Here's how the part is built. I have some questions about the finished solid (model axes, mm). Round coordinates to 2 decimals unless told otherwise and drop trailing zeros. Loops run counter-clockwise (first coordinate to the right, second up) from the corner with the lowest first, then second, coordinate; pieces in that order, holes last. Notation, with made-up numbers: M 26,1 L 41,1 A19 ccw 41,16 Z; hole C -14,-3.75 d10. An arc over 180 degrees is marked long. Answer as a JSON object with one key per item and string values.
from build123d import *

# Parameters (mm, degrees)
CYLINDER013_R           = 1.7
CYLINDER013_DEPTH       = 20
CYLINDER013_PITCH_ANGLE = 90
CYLINDER015_R           = 1.7
CYLINDER015_DEPTH       = 20
CYLINDER015_PITCH_ANGLE = 90
CYLINDER016_R           = 1.7
CYLINDER016_DEPTH       = 20
CYLINDER016_PITCH_ANGLE = 90
CYLINDER017_R           = 1.7
CYLINDER017_DEPTH       = 20
CYLINDER017_PITCH_ANGLE = 90
SKETCH013_W             = 400
SKETCH013_H             = 150
SKETCH013_R             = 1.7
SKETCH013_W_2           = 360
SKETCH013_H_2           = 70
PAD013_DEPTH            = 10


with BuildPart() as cylinder013:
    # Cylinder013 → Cylinder013 (new body)
    with BuildSketch(Plane.XY):
        Circle(CYLINDER013_R)
    extrude(amount=CYLINDER013_DEPTH)


with BuildPart() as cylinder013_1:
    # Cylinder013 pitch: moved
    add(cylinder013.part.rotate(Axis((0, 0, 0), (0, 1, 0)), CYLINDER013_PITCH_ANGLE))


with BuildPart() as cylinder013_2:
    # Cylinder013 placement: moved
    add(cylinder013_1.part.moved(Location((195, -65, 65))))


with BuildPart() as cylinder015:
    # Cylinder015 → Cylinder015 (new body)
    with BuildSketch(Plane.XY):
        Circle(CYLINDER015_R)
    extrude(amount=CYLINDER015_DEPTH)


with BuildPart() as cylinder015_1:
    # Cylinder015 pitch: moved
    add(cylinder015.part.rotate(Axis((0, 0, 0), (0, 1, 0)), CYLINDER015_PITCH_ANGLE))


with BuildPart() as cylinder015_2:
    # Cylinder015 placement: moved
    add(cylinder015_1.part.moved(Location((-215, -65, 65))))


with BuildPart() as cylinder016:
    # Cylinder016 → Cylinder016 (new body)
    with BuildSketch(Plane.XY):
        Circle(CYLINDER016_R)
    extrude(amount=CYLINDER016_DEPTH)


with BuildPart() as cylinder016_1:
    # Cylinder016 pitch: moved
    add(cylinder016.part.rotate(Axis((0, 0, 0), (0, 1, 0)), CYLINDER016_PITCH_ANGLE))


with BuildPart() as cylinder016_2:
    # Cylinder016 placement: moved
    add(cylinder016_1.part.moved(Location((-215, 45, 65))))


with BuildPart() as fusion004:
    # Cylinder017 → Cylinder017 (new body)
    with BuildSketch(Plane.XY):
        Circle(CYLINDER017_R)
    extrude(amount=CYLINDER017_DEPTH)


with BuildPart() as fusion004_1:
    # Cylinder017 pitch: moved
    add(fusion004.part.rotate(Axis((0, 0, 0), (0, 1, 0)), CYLINDER017_PITCH_ANGLE))


with BuildPart() as fusion004_2:
    # Cylinder017 placement: moved
    add(fusion004_1.part.moved(Location((195, 45, 65))))

    # Fusion004: union Cylinder013, Cylinder015, Cylinder016
    add(cylinder013_2.part)
    add(cylinder015_2.part)
    add(cylinder016_2.part)


with BuildPart() as cut016:
    # Sketch013 → Pad013 (new body)
    with BuildSketch(Plane(origin=(0, -10, 60), x_dir=(1, 0, 0), z_dir=(0, 0, 1))):
        Rectangle(SKETCH013_W, SKETCH013_H)
        with Locations((-170, 50)):
            Circle(SKETCH013_R, mode=Mode.SUBTRACT)
        with Locations((-170, -50)):
            Circle(SKETCH013_R, mode=Mode.SUBTRACT)
        with Locations((15, -50)):
            Circle(SKETCH013_R, mode=Mode.SUBTRACT)
        with Locations((170, -50)):
            Circle(SKETCH013_R, mode=Mode.SUBTRACT)
        with Locations((170, 50)):
            Circle(SKETCH013_R, mode=Mode.SUBTRACT)
        with Locations((15, 50)):
            Circle(SKETCH013_R, mode=Mode.SUBTRACT)
        Rectangle(SKETCH013_W_2, SKETCH013_H_2, mode=Mode.SUBTRACT)
    extrude(amount=PAD013_DEPTH)

    # Cut016: cut Fusion004
    add(fusion004_2.part, mode=Mode.SUBTRACT)


solid = cut016.part
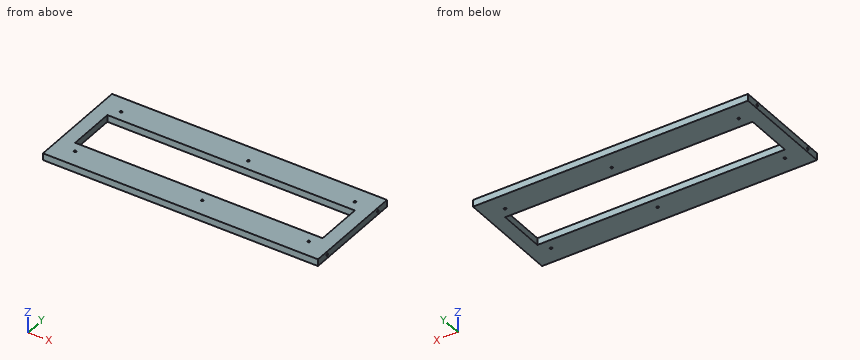
Item 1: I want a section at C-C, the plane z = 65. State how many separate pieces and enclosed holes the cut face has, then the cut area to 3 significant figures.
Resolved:
{"separate pieces": "1", "enclosed holes": "7", "area": "34,700 mm²"}
Item 2: I want a section at B-B, the plane y = -2. Please give me the cut outline in (x, z).
Resolved:
{"outline": "M -200,60 L -180,60 L -180,70 L -200,70 Z; M 180,60 L 200,60 L 200,70 L 180,70 Z"}
Item 3: I'm going to push flat-ended pins straight in: pin 1 Ø1 at (y, z) = (-65, 65) entering from -X; pin 2 Ø3 at (y, z) = (45, 65) entering from +X. Where does each tip first touch, or does it pass through?
Resolved:
{"pin 1": "x = -195", "pin 2": "x = 195"}
Item 4: Please list where these lines run through material, in increasing order: probe 1 along Y at (x, z) = (-170, 63); probe 2 along Y at (x, z) = (-196.45, 65); probe 3 along X at (y, z) = (-10, 66.25). Write a range as from..to.
Resolved:
{"probe 1": "-85..-61.7, -58.3..-45, 25..38.3, 41.7..65", "probe 2": "-85..-66.7, -63.3..43.3, 46.7..65", "probe 3": "-200..-180, 180..200"}
Item 5: I want a section at A-A, the plane x = -45. Please give me the cut outline in (y, z), then the cut area to 3 significant figures.
Resolved:
{"outline": "M -85,60 L -45,60 L -45,70 L -85,70 Z; M 25,60 L 65,60 L 65,70 L 25,70 Z", "area": "800 mm²"}
